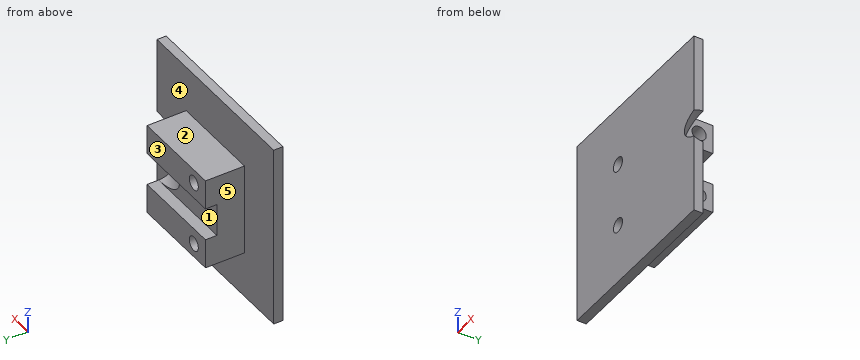
Autodesk Inventor part; units mm, degrees
ref_plane "Work Plane1" through (10, 8, 5) normal (0.866, -0.5, 0) x (0, 0, 1)
ref_plane "YZ Plane" through (0, 0, 0) normal (1, 0, 0) x (0, 1, 0)
ref_plane "XZ Plane" through (0, 0, 0) normal (0, 1, 0) x (-1, 0, 0)
sketch "Sketch1" plane through (0, 0, 0) normal (0, 1, 0) x (-1, 0, 0)
  line L0 (20, 20) -> (-20, 20)
  line L1 (-20, 20) -> (-20, -20)
  line L2 (-20, -20) -> (20, -20)
  line L3 (20, -20) -> (20, 20)
  point P0 (0, 0)
  dimension "d0" = 40
  dimension "d1" = 40
  dimension "d2" = 20
  dimension "d3" = 20
extrude "Extrusion1" add sketch "Sketch1" along normal blind 2
sketch "Sketch2" plane through (0, 2, 0) normal (0, 1, 0) x (1, 0, 0)
  line L0 (-10, -10) -> (10, -10)
  line L1 (10, -10) -> (10, 10)
  line L2 (10, 10) -> (-10, 10)
  line L3 (-10, 10) -> (-10, -10)
  point P0 (0, 0)
  dimension "d6" = 20
  dimension "d7" = 20
  dimension "d8" = 10
  dimension "d9" = 10
extrude "Extrusion2" add sketch "Sketch2" along normal blind 10
sketch "Sketch3" plane through (0, 12, 0) normal (0, 1, 0) x (1, 0, 0)
  line L0 (-10, 10) -> (-10, -10)
  line L1 (10, 10) -> (10, -10)
  line L2 (-10, -3.55) -> (10, -3.55)
  line L3 (10, -3.55) -> (10, 3.55)
  line L4 (10, 3.55) -> (-10, 3.55)
  line L5 (-10, 3.55) -> (-10, -3.55)
  point P0 (0, 0)
  point P1 (0, 3.55)
  point P2 (10, -3.55)
  dimension "d12" = 7.1
  dimension "d13" = 3.55
extrude "Extrusion3" cut sketch "Sketch3" against normal blind 4
ref_plane "Work Plane1" through (10, 8, 5) normal (0.866, -0.5, 0) x (0, 0, 1)
sketch "Sketch4" plane through (10, 8, 5) normal (0.866, -0.5, 0) x (0, 0, 1)
  line L0 (-1.45, 0) -> (-1.45, -3.4641)
  line L1 (-1.45, 10) -> (-8.55, 10)
  line L2 (-1.45, 0) -> (-1.45, 10)
  line L3 (-8.55, 0) -> (-1.45, 0)
  line L4 (-8.55, 10) -> (-8.55, 0)
  line L5 (-8.55, -3.4641) -> (-8.55, 0)
  circle A0 centre (-5, 0) radius 3.55
  point P0 (-5, 11.9282)
extrude "Extrusion4" cut sketch "Sketch4" along normal through all both and the other way through all contours A0 L3 | L3 A0
sketch "Sketch5" plane through (0, 12, 0) normal (0, 1, 0) x (1, 0, 0)
  line L0 (10, -10) -> (-10, -10)
  line L1 (10, -3.55) -> (-10, -3.55)
  line L2 (-10, -10) -> (10, -10)
  line L3 (10, -10) -> (10, -3.55)
  line L4 (10, -3.55) -> (-10, -3.55)
  line L5 (-10, -3.55) -> (-10, -10)
  line L6 (-10, 3.0802) -> (10, 3.0802)
  line L7 (10, 3.0802) -> (10, 10.1436)
  line L8 (10, 10.1436) -> (-10, 10.1436)
  line L9 (-10, 10.1436) -> (-10, 3.0802)
  point P0 (0, 0)
  point P1 (-10, -3.55)
extrude "Extrusion5" cut sketch "Sketch5" against normal blind 1.5
sketch "Sketch6" plane through (0, 10.5, 0) normal (0, 1, 0) x (1, 0, 0)
  circle A0 centre (-6, -7) radius 1.55
  circle A1 centre (-6, 7) radius 1.55
  line L0 (-10, 3.55) -> (-10, 10)
  line L1 (-10, -10) -> (-10, -3.55)
  line L2 (10, -10) -> (-10, -10)
  line L3 (-10, 10) -> (10, 10)
  point P0 (0, 0)
  point P1 (-10, -6.775)
  point P2 (-10, 3.5772)
  dimension "d21" = 3.1
  dimension "d22" = 3.1
  dimension "d23" = 4
  dimension "d24" = 4
  dimension "d25" = 3
  dimension "d26" = 3
extrude "Extrusion6" cut sketch "Sketch6" against normal through all
sketch "Sketch7" plane through (10, 2, 10) normal (1, 0, 0) x (0, 0, -1)
  circle A0 centre (3, 5.5) radius 1.55
  circle A1 centre (17, 5.5) radius 1.55
  line L0 (20, 0) -> (20, 8.5)
  line L1 (0, 0) -> (0, 8.5)
  line L2 (6.45, 8.5) -> (0, 8.5)
  line L3 (20, 8.5) -> (13.55, 8.5)
  point P0 (10, -2)
  point P1 (13.5772, 8.7)
  dimension "d29" = 3.1
  dimension "d30" = 3.1
  dimension "d31" = 3
  dimension "d32" = 3
  dimension "d33" = 3
  dimension "d34" = 3
extrude "Extrusion7" cut sketch "Sketch7" against normal blind 10
properties part number "Camera Holder 1"
Source: CAD feature listing. Evaluate the final solid. Frame: model axes, mm. Face numbers are marked on the shaded views. A direction names the side the tool comes from. Coordinates: 2 decimals unless noted, no trailing zeros. Loops run counter-clockwise (first coordinate to the right, second up) from the corner with the lowest first, then second, coordinate; pieces in that order, holes last. Notation, with made-up numbers: (86, -20) -> (130, -20) arc R9 cw to (130, -3) -> close; hole circle Ø7 at (-4.75, 69). An arc over 180 degrees is marked (long way). One line per item, written item: value. Start each with the question number.
Q1. Contact query for flat-ended pins moving along their axis: P1, Ø2.5, axis at y = 8, z = 7.5, coming from the +X side; P2, Ø2.5, axis at y = 7.5, z = -2, coming from the -X side; P3, Ø0.9, axis at y = 8, z = -6.5, coming from the +X side; P4, Ø1.9, axis at x = -6, z = -7, coming from the +Y side. Output: stop coordinate, or through.
Q2. Line query: line 1 along Z through (x, y) = (-6, 6.5); line 2 along X through (y, z) = (2.5, 7); line 3 along Y through (x, z) = (4, 7). Output: solid intervals per line, ascending.
Q3. Set-up query: the marked faces 1, 2, 3, 4 and 5. Return all of +Z, -Z, +X, -X, +Y, -Y with unobstructed straight access to the full face (end or side cutting, diameter ignored); none if empty.
Q4. Section query B-B, the plane z = -7. Return the cut outline in (x, y).
Q5. Section query A-A, the plane y = 2.5. Return the cut outline in (x, z), and give its area (3 significant figures).
Q6. Section query C-C, the plane x = -6. Return the cut outline in (y, z).
Q7. Section query D-D, the plane z = 4.5. Return the cut outline in (x, y).
Results:
1. P1: x = 10
1. P2: x = -10
1. P3: x = 0
1. P4: through
2. line 1: -10 to -8.55, -5.45 to 5.45, 8.55 to 10
2. line 2: -10 to -7.55, -4.45 to 10
2. line 3: 0 to 5.95, 9.05 to 10.5
3. face 1: +X, -X, +Y
3. face 2: +Z, +X, -X, +Y
3. face 3: +Z, -Z, +X, -X, +Y
3. face 4: +Y
3. face 5: +Z, -Z, -X, +Y
4. outline: (-20, 0) -> (-7.55, 0) -> (-7.55, 10.5) -> (-10, 10.5) -> (-10, 2) -> (-20, 2) -> close; (-4.45, 0) -> (20, 0) -> (20, 2) -> (10, 2) -> (10, 5.95) -> (0, 5.95) -> (0, 9.05) -> (10, 9.05) -> (10, 10.5) -> (-4.45, 10.5) -> close
5. outline: (-10, -10) -> (10, -10) -> (10, 10) -> (-10, 10) -> close; hole circle Ø3.1 at (-6, -7); hole circle Ø3.1 at (-6, 7)
5. area: 385 mm^2
6. outline: (0, -20) -> (2, -20) -> (2, -10) -> (10.5, -10) -> (10.5, -8.55) -> (0, -8.55) -> close; (0, -5.45) -> (10.5, -5.45) -> (10.5, -3.55) -> (8, -3.55) -> (8, 3.55) -> (10.5, 3.55) -> (10.5, 5.45) -> (0, 5.45) -> close; (0, 8.55) -> (10.5, 8.55) -> (10.5, 10) -> (2, 10) -> (2, 20) -> (0, 20) -> close
7. outline: (-20, 0) -> (20, 0) -> (20, 2) -> (10, 2) -> (10, 10.5) -> (-10, 10.5) -> (-10, 2) -> (-20, 2) -> close
